Can you work these out from the model? Positions are in its coordinate system, mm. A direction names the side the tool comes from. Give positions to 0.01 mm unless a question says otherwise; leave off trailing zeros. Order: outer loops, then holes, each group sorted by start corner. A loop starts at its lowest first (then second) coordinate and runs counter-clockwise, first axis right, second up. Notation, with made-up numbers: M 35,87.5 L 43,87.5 A12 ccw 43,107.5 Z; hole C 76,-14 d6. An arc over 180 degrees is marked long. Write each question's results on one line, items separated by ' | '.
from build123d import *

# Parameters (mm, degrees)
F1_DEPTH = 60
F3_D     = 8.8
F3_DEPTH = 10
F3_TIP   = 2.6437867237


with BuildPart() as f1:
    # F0 (on Front) → F1 (new body)
    with BuildSketch(Plane.XZ):
        Polygon((-3.7746716016, 2.5), (-3.7746716016, 0), (3.7253283984, 0), (3.7253283984, 2.5), (7.4753283984, 2.5), (7.4753283984, 4), (3.7253283984, 7.5), (-3.7746716016, 7.5), (-7.5246716016, 4), (-7.5246716016, 2.5), align=None)
        Polygon((3.7253283984, 0), (-3.7746716016, 0), (-7.5246716016, 0), (-7.5246716016, -10), (22.4753283984, -10), (22.4753283984, 0), align=None)
    extrude(amount=F1_DEPTH)

    # F3
    with Locations(Plane.YZ.offset(22.4753283984)):
        with Locations((-50, -5), (-10, -5)):
            Hole(F3_D / 2, depth=F3_DEPTH)
            with Locations((0, 0, -(F3_DEPTH + F3_TIP / 2))):  # 118° drill point
                Cone(0, F3_D / 2, F3_TIP, mode=Mode.SUBTRACT)


solid = f1.part
(1) Imagine slicing it at A-A, the plane x = 14. Write out the boundary of the cut face in (y, z).
Data:
outline: M -60,-10 L 0,-10 L 0,0 L -60,0 Z; hole C -50,-5 d8.8; hole C -10,-5 d8.8
(2) For faces 4 (the face through (-7.525, -30, -5)), 5 (the face through (-6, -30, 2.5)), 6 (the face through (-5.623, -29.58, 5.774)), 7 (the face through (6, -30, 2.5)), 8 (the face through (17.405, -14.197, -3.678)), which set-ups out of +Z, -Z, +X, -X, +Y, -Y let a thin tool reach every point of the face, with its end or its side?
Data:
face 4: +Z, -Z, -X, +Y, -Y | face 5: -X, +Y, -Y | face 6: +Z, -X, +Y, -Y | face 7: +X, +Y, -Y | face 8: +X
(3) Imagine slicing it at C-C, the plane x = 5.5. Write out the boundary of the cut face in (y, z), plus the area to 3 significant figures.
Data:
outline: M -60,-10 L 0,-10 L 0,0 L -60,0 Z; M -60,2.5 L 0,2.5 L 0,5.84 L -60,5.84 Z | area: 801 mm2
(4) Imagine slicing it at B-B, the plane y = -25. Write out the boundary of the cut face in (x, z).
Data:
outline: M -7.52,-10 L 22.48,-10 L 22.48,0 L 3.73,0 L 3.73,2.5 L 7.48,2.5 L 7.48,4 L 3.73,7.5 L -3.77,7.5 L -7.52,4 L -7.52,2.5 L -3.77,2.5 L -3.77,0 L -7.52,0 Z
(5) Will these pins go through, and if not, where does the flat tip stop? P1, Ø1.5, axis at y = -16, z = 5.5, coming from the -X side; P2, Ø4, axis at x = -6.5, y = -32, coming from the +Z side; P3, Ø8, axis at y = -50, z = -5, coming from the +X side (3 decimals).
Data:
P1: stops at x = -6.72 | P2: stops at z = 6.82 | P3: stops at x = 12.235
(6) I need wall thicknesses on L1, parallel to Y at x = 19.25, z = -5; L2, parallel to Z at x = 19, y = -50; L3, parallel to Z at x = 18, y = -5.5. Which ranges of each line are inside material? Lowest first, please. Write a range as from..to.
Data:
L1: y = -60..-54.4, -45.6..-14.4, -5.6..0 | L2: z = -10..-9.4, -0.6..0 | L3: z = -10..0
(7) We'd pull the mould along Z, two halves only. Please class faces 1 (the face through (17.405, -54.197, -3.678)), 2 (the face through (5.627, -29.58, 5.726)), 3 (the face through (7.475, -30, 3)): +Z half, -Z half, draft (parallel to the pull), parting line (faces both ways), or undercut.
Data:
face 1: undercut | face 2: +Z half | face 3: draft
